Could you check a few things on this model? Use its own coordinates, in mm. A direction names the side the tool comes from. Coordinates: 2 decimals unless noted, no trailing zeros. Loops run counter-clockwise (first coordinate to the right, second up) from the corner with the lowest first, then second, coordinate; pieces in that order, holes last. Notation, with made-up numbers: M 75.5,26 L 120.5,26 A35 cw 120.5,64 Z; hole C 3.25,35.25 d2. An arc over 180 degrees is marked long. Write each question's results on one line, items separated by ' | '.
```python
from build123d import *

# Parameters (mm, degrees)
BOSS_EXTRUDE1_DEPTH = 101.6
SKETCH2_R           = 2.1844
SKETCH2_R_2         = 40.005
CUT_EXTRUDE1_DEPTH  = 136.951937251
FILLET1_R           = 2.54
FILLET2_R           = 1.27


with BuildPart() as part:
    # Sketch1 → Boss-Extrude1 (new body)
    with BuildSketch(Plane.XY):
        Polygon((85.725, 0), (-85.725, 0), (-87.558087105, -3.175), (-54.56251922, -22.225), (-52.3875, -22.225), (-52.3875, -6.35), (52.3875, -6.35), (52.3875, -22.225), (54.56251922, -22.225), (87.558087105, -3.175), align=None)
    extrude(amount=BOSS_EXTRUDE1_DEPTH)

    # Sketch2 → Cut-Extrude1 (cut, through all)
    with BuildSketch(Plane(origin=(0, 0, 0), x_dir=(1, 0, 0), z_dir=(0, 1, 0))):
        with Locations(Location((77.75575, -90.805, 0), (0, 0, 180))):
            Circle(SKETCH2_R)
        with Locations(Location((-77.75575, -90.805, 0), (0, 0, 180))):
            Circle(SKETCH2_R)
        with Locations(Location((-77.75575, -10.795, 0), (0, 0, 180))):
            Circle(SKETCH2_R)
        with Locations((77.75575, -10.795)):
            Circle(SKETCH2_R)
        with Locations(Location((0, -50.8, 0), (0, 0, 180))):
            Circle(SKETCH2_R_2)
    extrude(amount=-CUT_EXTRUDE1_DEPTH, mode=Mode.SUBTRACT)

    # Fillet1
    fillet1_edges = [part.edges().sort_by_distance(p)[0] for p in [
        (87.558087105, -3.175, 50.8),
        (52.3875, -6.35, 50.8),
        (-52.3875, -6.35, 50.8),
        (-87.558087105, -3.175, 50.8),
    ]]
    fillet(fillet1_edges, radius=FILLET1_R)

    # Fillet2
    fillet2_edges = [part.edges().sort_by_distance(p)[0] for p in [
        (54.56251922, -22.225, 50.8),
        (52.3875, -22.225, 50.8),
        (-52.3875, -22.225, 50.8),
        (-54.56251922, -22.225, 50.8),
    ]]
    fillet(fillet2_edges, radius=FILLET2_R)


solid = part.part
```
(1) Imagine slicing it at B-B, the plane x = 0. List the corners of the cut face in (y, z) for me (3 decimals).
Reported:
outline: M -6.35,0 L 0,0 L 0,10.795 L -6.35,10.795 Z; M -6.35,90.805 L 0,90.805 L 0,101.6 L -6.35,101.6 Z
(2) Imagine slicing it at C-C, the plane y = -15.75. List the corners of the cut face in (x, z) for me, and give its area (3 significant figures).
Reported:
outline: M -65.78,0 L -52.39,0 L -52.39,101.6 L -65.78,101.6 Z; M 52.39,0 L 65.78,0 L 65.78,101.6 L 52.39,101.6 Z | area: 2,720 mm2
(3) If we mould it in two halves opening along Z, with no side actions, what happens to faces 1 (the cylindrical face through (75.67, -4.98, 91.46)), 2 (the flat face through (-1, -6, 101.6)), 3 (the cylindrical face through (-75.573, -3.901, 10.891)), 4 (the flat face through (69.894, -13.373, 50.089))? For each: released by +Z, released by -Z, zero draft, split by the parting line, or undercut.
Reported:
face 1: undercut | face 2: released by +Z | face 3: undercut | face 4: zero draft
(4) Which directions (+Z, -Z, +X, -X, +Y, -Y) give clear straight access to the entire face, cutting with the end or side of a thin tool? Please do faces 5 (the flat face through (52.388, -15, 50)), 6 (the flat face through (-1, -6, 0)).
Reported:
face 5: +Z, -Z, -Y | face 6: -Z, +X, -X, +Y, -Y
(5) Please list where these lines run through material, in increasing order: probe 1 along Z at (x, y) = (0, -3.25) (3 decimals); probe 2 along X at (y, z) = (-13, 19); probe 3 along X at (y, z) = (-16.75, 25.5). Write a range as from..to.
Reported:
probe 1: z = 0..10.795, 90.805..101.6 | probe 2: x = -70.54..-52.39, 52.39..70.54 | probe 3: x = -64.05..-52.39, 52.39..64.05
(6) Will these pins go through, and if not, where does the flat tip stop? P1, Ø1.5, axis at y = -10, z = 30.5, coming from the +X side; P2, Ø5, axis at y = -6, z = 85.5, coming from the +X side; P3, Ø5.5, axis at x = -77.76, z = 10.8, coming from the -Y side.
Reported:
P1: stops at x = 77.04 | P2: stops at x = 86.3 | P3: stops at y = -10.42
